Source: CAD feature listing. Evaluate the final solid. Frame: model axes, mm. A direction names the side the tool comes from. Give positions to 0.01 mm unless a question says otherwise; leave off trailing zeros. Order: outer loops, then holes, each group sorted by start corner. A loop starts at its lowest first (then second) coordinate and runs counter-clockwise, first axis right, second up. Notation, with made-up numbers: M 27.25,68.25 L 32.25,68.25 A23 cw 32.25,96.25 Z; hole C 70.5,42 d11. An arc over 180 degrees is marked long. Answer as a JSON object with one key per item and string values. Group by question number.
1. Pin query (flat end, axial travel): P1, Ø0.9, axis at y = -4.5, z = 1.5, coming from the +X side. Return the tip coordinate at first contact, or that it passes through.
2. Section query B-B (x = -9). Output: boundary loops of the cut face in (y, z).
3. Section query A-A (z = 2.3). Output: boundary loops of the cut face in (x, y), plus the area to 3 significant figures.
4. Material intervals for L1, parallel to Y at x = 2.5, z = 2.5; L2, parallel to Y at x = -32, z = 1.1; L3, parallel to X at y = 43, z = 0.8, sorted ascending. Write a range as [from, to].
5. Section query C-C (x = -27). Output: boundary loops of the cut face in (y, z), plus the area to 3 significant figures.
6. Pull-direction query (X, two-part tool) for faces 4 (the flat face through (9, 22, 3)), 5 (the flat face through (-11.96, -4, 1)), 6 (the cylindrical face through (-30.946, 42.915, 1.479)); classes: +X half, -X half, draft (parallel to the pull), parting line (faces both ways), or undercut.
7. Set-up query: faces 1 (the flat face through (18.04, -4, 1)), 2 (the flat face through (-36.96, 11, 1)), 3 (the flat face through (43.04, -4, 1)). Return all of +Z, -Z, +X, -X, +Y, -Y with unobstructed straight access to the full face (end or side cutting, diameter ignored); none if empty.
from build123d import *

# Parameters (mm, degrees)
RESSALTO_EXTRUS_O1_DEPTH = 3


with BuildPart() as part:
    # Esboço1 → Ressalto-extrusão1 (new body)
    with BuildSketch(Plane.XY):
        with BuildLine():
            Line((43.040081042, -1.381695114), (56.040081042, -1.381695114))
            Line((56.040081042, -1.381695114), (56.040081042, 28.618304886))
            ThreePointArc((56.040081042, 28.618304886), (50.182216666, 42.76044051), (36.040081042, 48.618304886))
            Line((36.040081042, 48.618304886), (-16.959918958, 48.618304886))
            ThreePointArc((-16.959918958, 48.618304886), (-31.102054581, 42.76044051), (-36.959918958, 28.618304886))
            Line((-36.959918958, 28.618304886), (-36.959918958, -1.381695114))
            Line((-36.959918958, -1.381695114), (-36.959918958, -6.381695114))
            Line((-36.959918958, -6.381695114), (-11.959918958, -6.381695114))
            Line((-11.959918958, -6.381695114), (-11.959918958, -1.381695114))
            Line((-11.959918958, -1.381695114), (18.040081042, -1.381695114))
            Line((18.040081042, -1.381695114), (18.040081042, -6.381695114))
            Line((18.040081042, -6.381695114), (43.040081042, -6.381695114))
            Line((43.040081042, -6.381695114), (43.040081042, -1.381695114))
        make_face()
    extrude(amount=RESSALTO_EXTRUS_O1_DEPTH)


solid = part.part
Answer sheet:
{
 "1": {"P1": "x = 43.04"},
 "2": {"outline": "M -1.38,0 L 48.62,0 L 48.62,3 L -1.38,3 Z"},
 "3": {"outline": "M -36.96,-6.38 L -11.96,-6.38 L -11.96,-1.38 L 18.04,-1.38 L 18.04,-6.38 L 43.04,-6.38 L 43.04,-1.38 L 56.04,-1.38 L 56.04,28.62 A20 ccw 36.04,48.62 L -16.96,48.62 A20 ccw -36.96,28.62 Z", "area": "4,730 mm^2"},
 "4": {"L1": "[-1.38, 48.62]", "L2": "[-6.38, 41.8]", "L3": "[-30.86, 49.94]"},
 "5": {"outline": "M -6.38,0 L 45.92,0 L 45.92,3 L -6.38,3 Z", "area": "157 mm^2"},
 "6": {"face 4": "draft", "face 5": "undercut", "face 6": "-X half"},
 "7": {"face 1": "+Z, -Z, -Y", "face 2": "+Z, -Z, -X, +Y, -Y", "face 3": "+Z, -Z, +X, -Y"}
}
